Model file for the job. Use its own axes, mm. Face numbers are marked on the shaded views. A direction names the side the tool comes from. Give positions to 0.01 mm unless a question says otherwise; leave off trailing zeros. Loops run counter-clockwise (first coordinate to the right, second up) from the corner with the lowest first, then second, coordinate; pieces in that order, holes last. Notation, with made-up numbers: (62, 79.25) - (109, 79.25) arc R22 cw to (109, 108.25) - close; hole circle Ø2 at (50, 52). An arc over 180 degrees is marked (long way). Use a Markdown table: item, result.
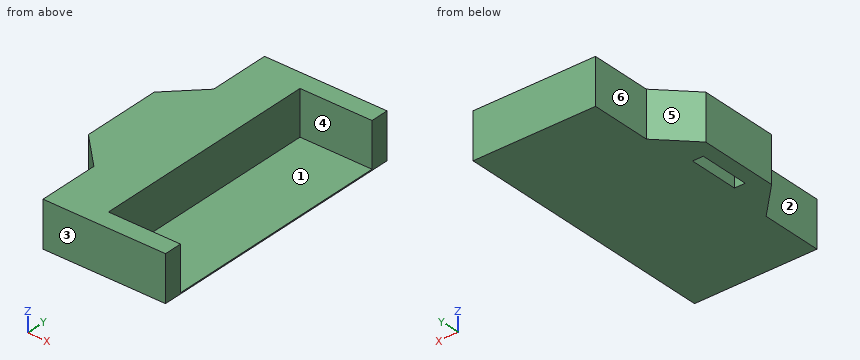
from build123d import *

# Parameters (mm, degrees)
F0_W     = 1.905
F0_H     = 8.89
F1_DEPTH = 7.62
F3_DEPTH = 0.4
F4_W     = 12.7
F4_H     = 40.64
F5_DEPTH = 0.2
F6_SIZE  = 5.71499


# Not quite as in the source:
# - a fillet or chamfer is up to 0.001 mm smaller than in the source, because OpenCascade refuses the exact size


with BuildPart() as f1:
    # F0 (on Top) → F1 (new body)
    with BuildSketch(Plane.XY):
        Polygon((-14.605, 6.985), (-14.605, 0), (-14.605, -6.985), (-8.89, -6.985), (-8.89, -23.495), (12.7, -23.495), (12.7, -20.32), (0, -20.32), (0, 0), (0, 20.32), (12.7, 20.32), (12.7, 23.495), (-8.89, 23.495), (-8.89, 6.985), align=None)
        with Locations((-11.1125, 0)):
            Rectangle(F0_W, F0_H, mode=Mode.SUBTRACT)
    extrude(amount=F1_DEPTH)

    # F2 (on face) → F3 (join)
    with BuildSketch(Plane.XY.offset(7.62)):
        Polygon((0, -20.32), (0, 20.32), (12.7, 20.32), (12.7, 23.495), (-8.89, 23.495), (-8.89, 6.985), (-14.605, 6.985), (-14.605, -6.985), (-8.89, -6.985), (-8.89, -23.495), (12.7, -23.495), (12.7, -20.32), align=None)
    extrude(amount=F3_DEPTH)

    # F4 (on face) → F5 (join)
    with BuildSketch(Plane(origin=(0, 0, 0), x_dir=(1, 0, 0), z_dir=(0, 0, -1))):
        with Locations((6.35, 0)):
            Rectangle(F4_W, F4_H)
    extrude(amount=-F5_DEPTH)

    # F6 (size 5.715 in the source; OpenCascade refuses exactly that, so slightly less here)
    f6_edges = [f1.edges().sort_by_distance(p)[0] for p in [
        (-8.89, 6.985, 4.01),
        (-8.89, -6.985, 4.01),
    ]]
    chamfer(f6_edges, length=F6_SIZE)


solid = f1.part
(1) Drill centre lines: probe 1 along Y at (x, z) = (6, 7) (3 decimals); probe 2 along X at (y, z) = (-4, 2.5) (3 decimals); probe 3 along X at (y, z) = (20.5, 0.75). Where is each one in solid material? Low to high. Write a range as [from, to].
Computed:
| item | result |
|---|---|
| probe 1 | [-23.495, -20.32], [20.32, 23.495] |
| probe 2 | [-14.605, -12.065], [-10.16, 0] |
| probe 3 | [-8.89, 12.7] |
(2) 3-axis set-ups, long thin cutter, end or side, ignore diameter. For the marked faces 1, 2 and 3: which of +Z, -Z, +X, -X, +Y, -Y reach the whole face in a straight line?
Computed:
| item | result |
|---|---|
| face 1 | +Z, +X |
| face 2 | +Z, -Z, -X, -Y |
| face 3 | +Z, -Z, +X, -X, -Y |
(3) Mould opens along Y. For the marked faces 4, 5 and 6 say: pulls with the +Y half, pulls with the -Y half, needs draft (parallel to the pull), parting line crosses it, or undercut.
Computed:
| item | result |
|---|---|
| face 4 | undercut |
| face 5 | pulls with the +Y half |
| face 6 | needs draft |
(4) Slice it at D-D, the plane x = -11.25. Write the cut outline in (y, z) (3 decimals), plus the area to 3 significant figures.
Computed:
| item | result |
|---|---|
| outline | (-10.34, 0) - (-4.445, 0) - (-4.445, 7.62) - (4.445, 7.62) - (4.445, 0) - (10.34, 0) - (10.34, 8.02) - (-10.34, 8.02) - close |
| area | 98.1 mm² |
(5) Slice it at A-A, the plane y = 3. Write the cut outline in (x, z) (3 decimals), plus the area to 3 significant figures.
Computed:
| item | result |
|---|---|
| outline | (-14.605, 0) - (-12.065, 0) - (-12.065, 7.62) - (-10.16, 7.62) - (-10.16, 0) - (12.7, 0) - (12.7, 0.2) - (0, 0.2) - (0, 8.02) - (-14.605, 8.02) - close |
| area | 105 mm² |
(6) Pin check, flat tips, straight feed: P1, Ø2, axis at x = 6, y = -12.5, coming from the +Z side; P2, Ø2.5, axis at y = 1, z = 4, coming from the +X side; P3, Ø2, axis at y = -17, z = 6.5, coming from the -X side. Stop position of each tip, or through.
Computed:
| item | result |
|---|---|
| P1 | z = 0.2 |
| P2 | x = 0 |
| P3 | x = -8.89 |
(7) Slice it at C-C, the plane x = 2.25. Write the cut outline in (y, z) (3 decimals), plus the area to 3 significant figures.
Computed:
| item | result |
|---|---|
| outline | (-23.495, 0) - (23.495, 0) - (23.495, 8.02) - (20.32, 8.02) - (20.32, 0.2) - (-20.32, 0.2) - (-20.32, 8.02) - (-23.495, 8.02) - close |
| area | 59.1 mm² |
